Model file for the job. Use its own axes, mm. Give positions to 0.01 mm unless a question says otherwise; leave off trailing zeros. Loops run counter-clockwise (first coordinate to the right, second up) from the corner with the lowest first, then second, coordinate; pieces in that order, holes last. Notation, with made-up numbers: (-10.5, 61) - (18.5, 61) arc R14 ccw to (18.5, 83) - close; hole circle Ø7 at (21, 89.5). An arc over 180 degrees is marked (long way). Use a Markdown table: item, result.
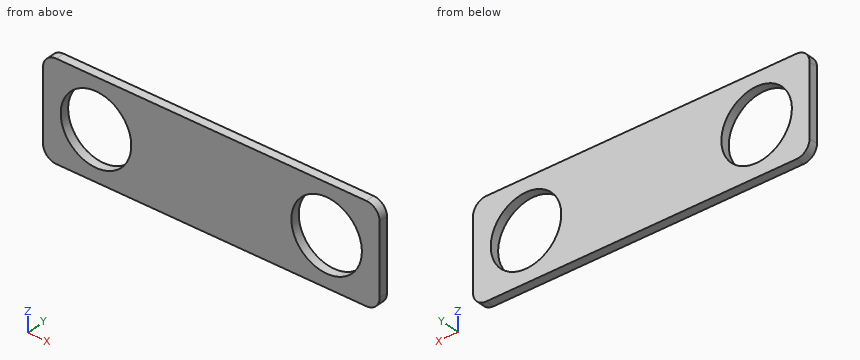
from build123d import *

# Parameters (mm, degrees)
SKETCH1_W           = 75.9
SKETCH1_H           = 21.9
SKETCH1_R           = 7.95
BOSS_EXTRUDE1_DEPTH = 2
FILLET1_R           = 3


with BuildPart() as part:
    # Sketch1 → Boss-Extrude1 (new body)
    with BuildSketch(Plane(origin=(0, 0, 0), x_dir=(1, 0, 0), z_dir=(0, 1, 0))):
        Rectangle(SKETCH1_W, SKETCH1_H)
        with Locations(Location((26, 0, 0), (0, 0, 270))):
            Circle(SKETCH1_R, mode=Mode.SUBTRACT)
        with Locations(Location((-26, 0, 0), (0, 0, 270))):
            Circle(SKETCH1_R, mode=Mode.SUBTRACT)
    extrude(amount=BOSS_EXTRUDE1_DEPTH)

    # Fillet1
    fillet1_edges = [part.edges().sort_by_distance(p)[0] for p in [
        (37.95, 1, -10.95),
        (37.95, 1, 10.95),
        (-37.95, 1, 10.95),
        (-37.95, 1, -10.95),
    ]]
    fillet(fillet1_edges, radius=FILLET1_R)


solid = part.part
(1) Slice it at C-C, the plane y = 1. Write the cut outline in (x, z).
Computed:
| item | result |
|---|---|
| outline | (-37.95, -7.95) arc R3 ccw to (-34.95, -10.95) - (34.95, -10.95) arc R3 ccw to (37.95, -7.95) - (37.95, 7.95) arc R3 ccw to (34.95, 10.95) - (-34.95, 10.95) arc R3 ccw to (-37.95, 7.95) - close; hole circle Ø15.9 at (-26, 0); hole circle Ø15.9 at (26, 0) |
(2) Slice it at B-B, the plane x = 26. Write the cut outline in (y, z), plus the area to 3 significant figures.
Computed:
| item | result |
|---|---|
| outline | (0, -10.95) - (2, -10.95) - (2, -7.95) - (0, -7.95) - close; (0, 7.95) - (2, 7.95) - (2, 10.95) - (0, 10.95) - close |
| area | 12.0 mm² |
(3) Slice it at D-D, the plane z = 0. Write the cut outline in (x, y), plus the area to 3 significant figures.
Computed:
| item | result |
|---|---|
| outline | (-37.95, 0) - (-33.95, 0) - (-33.95, 2) - (-37.95, 2) - close; (-18.05, 0) - (18.05, 0) - (18.05, 2) - (-18.05, 2) - close; (33.95, 0) - (37.95, 0) - (37.95, 2) - (33.95, 2) - close |
| area | 88.2 mm² |
(4) Slice it at A-A, the plane z = 5.75. Write the cut outline in (x, y), plus the area to 3 significant figures.
Computed:
| item | result |
|---|---|
| outline | (-37.95, 0) - (-31.49, 0) - (-31.49, 2) - (-37.95, 2) - close; (-20.51, 0) - (20.51, 0) - (20.51, 2) - (-20.51, 2) - close; (31.49, 0) - (37.95, 0) - (37.95, 2) - (31.49, 2) - close |
| area | 108 mm² |
(5) Drill centre lines: probe 1 along X at (y, z) = (1, 0); probe 2 along X at (y, z) = (0.6, 6.25); probe 3 along Z at (x, y) = (32, 0.45). Where is each one in solid material? Low to high. Write a range as [from, to].
Computed:
| item | result |
|---|---|
| probe 1 | [-37.95, -33.95], [-18.05, 18.05], [33.95, 37.95] |
| probe 2 | [-37.95, -30.91], [-21.09, 21.09], [30.91, 37.95] |
| probe 3 | [-10.95, -5.22], [5.22, 10.95] |
